Input: dimensioned drawing with shaded views. Units: mm. Origin: part minimum x, y, z. A direction names the side the tool comes from. Give positions to 0.01 mm unless a question says otherwise; leave off trailing zeros. Write each loop counter-clockwise with the first axis right and the second up, starting at its lowest first coordinate (ties: lowest second). Pieces come first, ordered by that corner, then holes. Notation, with made-up numbers: (-4, -17) -> (0, -17) arc R29 cw to (0, 5) -> close; hole circle Ø7 at (-8.5, 40). An arc over 180 degrees is marked (long way). Return JSON: item names as keys, results as strings. Group by question number.
Item 1: Set-up query: the marked faces 1 and 2. Return all of +Z, -Z, +X, -X, +Y, -Y with unobstructed straight access to the full face (end or side cutting, diameter ignored); none if empty.
Item 2: Line query: line 1 (X direction, y = 5.25, z = 38.1); line 2 (Z direction, x = 22.5, y = 6); line 3 (Y direction, x = 46, z = 25). Output: solid intervals per line, ascending. Write a range as [from, to].
Item 3: Section C-C, the plane y = 8.5. Return loops of the section in (x, z).
Item 4: Pin query (flat end, axial travel): P1, Ø4, axis at x = 20.64, z = 38.1, coming from the +Y side (3 decimals); P2, Ø3, axis at x = 15, z = 15.5, coming from the -Y side; P3, Ø20.5, axis at y = 33, z = 24, coming from the -X side; P4, Ø4, axis at y = 9, z = 38, coming from the -X side. Return the tip coordinate at first contact, or that it passes through.
Item 5: Mould query, pull axis Z, two halves, no side actions, for the marked faces 3, 4, 5 and 6. Classes: released by +Z, released by -Z, zero draft, split by the parting line, or undercut.
Item 6: Section B-B, the plane x = 46. Return loops of the section in (y, z) (1 decimal).
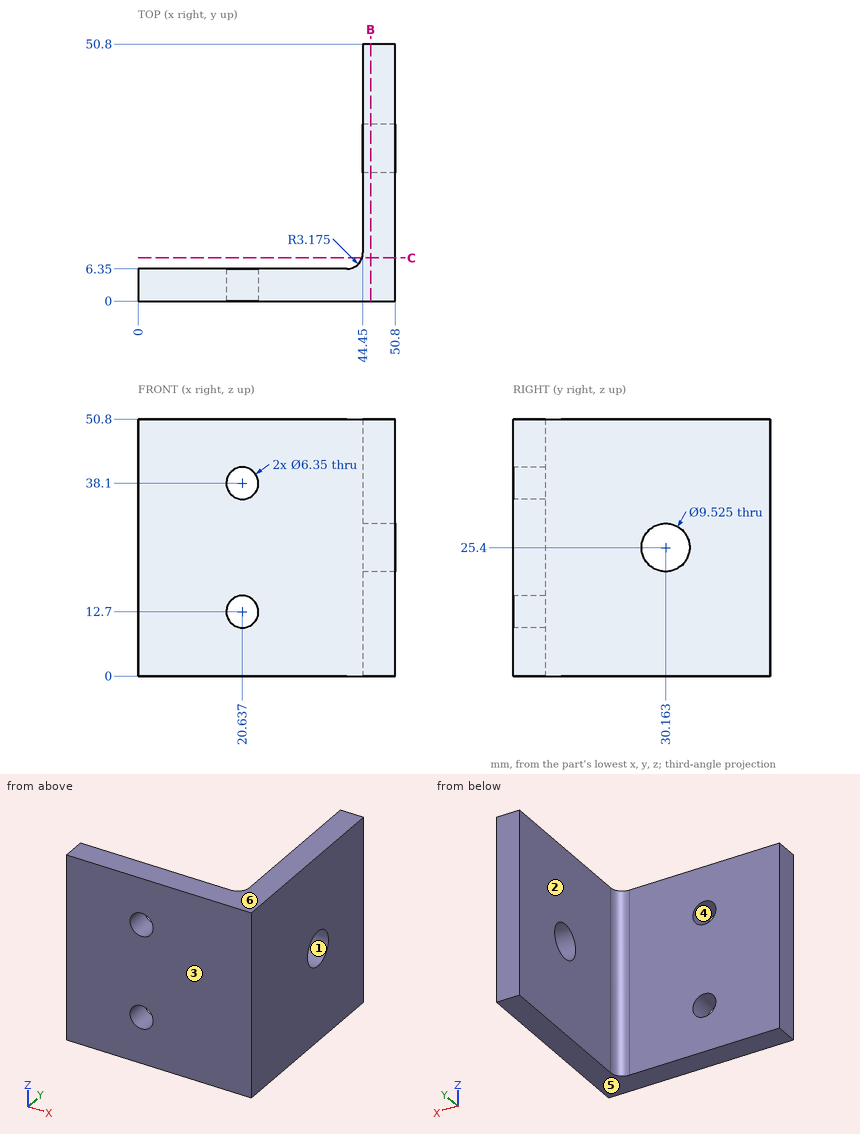
Answer below:
{
 "1": {"face 1": "+X, -X", "face 2": "+Z, -Z, -X, +Y"},
 "2": {"line 1": "x = [0, 17.46], [23.81, 50.8]", "line 2": "z = [0, 10.13], [15.27, 35.53], [40.67, 50.8]", "line 3": "y = [0, 25.42], [34.91, 50.8]"},
 "3": {"outline": "(44.28, 0) -> (50.8, 0) -> (50.8, 50.8) -> (44.28, 50.8) -> close"},
 "4": {"P1": "passes through", "P2": "stops at y = 0", "P3": "stops at x = 44.45", "P4": "stops at x = 43.2"},
 "5": {"face 3": "zero draft", "face 4": "undercut", "face 5": "released by -Z", "face 6": "released by +Z"},
 "6": {"outline": "(0, 0) -> (50.8, 0) -> (50.8, 50.8) -> (0, 50.8) -> close; hole circle Ø9.5 at (30.2, 25.4)"}
}
